Part model, mm, in its own coordinate system. A direction names the side the tool comes from. Give positions to 0.01 mm unless a question says otherwise; leave off trailing zeros. Order: outer loops, then holes, each group sorted by start corner. A loop starts at its lowest first (then second) coordinate and runs counter-clockwise, first axis right, second up. Notation, with made-up numbers: (66.25, 74) - (115.25, 74) arc R37 cw to (115.25, 111) - close; hole circle Ø4 at (86.5, 81). An arc over 180 degrees is marked (long way). One line per item, written item: value.
```python
from build123d import *

# Parameters (mm, degrees)
SKETCH1_W           = 2.4
SKETCH1_H           = 20
SKETCH1_H_2         = 2.4
SKETCH1_W_2         = 20
BOSS_EXTRUDE1_DEPTH = 20
BOSS_EXTRUDE2_DEPTH = 2.4
CUT_EXTRUDE1_REACH  = 4.4
SKETCH4_R           = 1.75
CUT_EXTRUDE2_REACH  = 4.4
SKETCH5_R           = 1.75
CUT_EXTRUDE3_REACH  = 24.4
SKETCH6_R           = 1.75
SKETCH7_R           = 2
BOSS_EXTRUDE3_DEPTH = 5
FILLET1_R           = 5


with BuildPart() as part:
    # Sketch1 → Boss-Extrude1 (new body)
    with BuildSketch(Plane(origin=(0, 0, 0), x_dir=(1, 0, 0), z_dir=(0, 1, 0))):
        with Locations((-1.2, 10)):
            Rectangle(SKETCH1_W, SKETCH1_H)
        with Locations((-1.2, -1.2)):
            Rectangle(SKETCH1_W, SKETCH1_H_2)
        with Locations((10, -1.2)):
            Rectangle(SKETCH1_W_2, SKETCH1_H_2)
    extrude(amount=-BOSS_EXTRUDE1_DEPTH)

    # Sketch2 → Boss-Extrude2 (add)
    with BuildSketch(Plane(origin=(0, 0, 0), x_dir=(1, 0, 0), z_dir=(0, 1, 0))):
        Polygon((20, -2.4), (20, 40), (0, 40), (0, 20), (-2.4, 20), (-2.4, -2.4), align=None)
    extrude(amount=BOSS_EXTRUDE2_DEPTH)

    # Sketch4 → Cut-Extrude1 (cut, up to next)
    with BuildSketch(Plane(origin=(0, 0, 0), x_dir=(0, 0, -1), z_dir=(1, 0, 0)), mode=Mode.PRIVATE) as cut_extrude1_sk1:
        with Locations((10, -10)):
            Circle(SKETCH4_R)
    cut_extrude1_tool1 = extrude(cut_extrude1_sk1.sketch, amount=-CUT_EXTRUDE1_REACH, mode=Mode.PRIVATE) & part.part
    add(cut_extrude1_tool1.solids().sort_by_distance((0, -10, -10))[0], mode=Mode.SUBTRACT)

    # Sketch5 → Cut-Extrude2 (cut, up to next)
    with BuildSketch(Plane(origin=(0, 0, 0), x_dir=(-1, 0, 0), z_dir=(0, 0, -1)), mode=Mode.PRIVATE) as cut_extrude2_sk1:
        with Locations((-10, -10)):
            Circle(SKETCH5_R)
    cut_extrude2_tool1 = extrude(cut_extrude2_sk1.sketch, amount=-CUT_EXTRUDE2_REACH, mode=Mode.PRIVATE) & part.part
    add(cut_extrude2_tool1.solids().sort_by_distance((10, -10, 0))[0], mode=Mode.SUBTRACT)

    # Sketch6 → Cut-Extrude3 (cut, up to next)
    with BuildSketch(Plane(origin=(0, 2.4, 0), x_dir=(1, 0, 0), z_dir=(0, 1, 0)), mode=Mode.PRIVATE) as cut_extrude3_sk1:
        with Locations((10, 30)):
            Circle(SKETCH6_R)
    cut_extrude3_tool1 = extrude(cut_extrude3_sk1.sketch, amount=-CUT_EXTRUDE3_REACH, mode=Mode.PRIVATE) & part.part
    add(cut_extrude3_tool1.solids().sort_by_distance((10, 2.4, -30))[0], mode=Mode.SUBTRACT)

    # Sketch7 → Boss-Extrude3 (add)
    with BuildSketch(Plane.XZ):
        with Locations((10, -10)):
            Circle(SKETCH7_R)
    extrude(amount=BOSS_EXTRUDE3_DEPTH)

    # Fillet1
    fillet1_edges = [part.edges().sort_by_distance(p)[0] for p in [
        (20, -20, 1.2),
        (20, 1.2, -40),
        (0, 1.2, -40),
        (-1.2, -20, -20),
    ]]
    fillet(fillet1_edges, radius=FILLET1_R)


solid = part.part
```
1) Cut at A-A, the plane y = -10. Give the cut face in (x, z), then the cut area to 3 significant figures.
Outcome:
outline: (-2.4, -20) - (0, -20) - (0, -11.75) - (-2.4, -11.75) - close; (-2.4, -8.25) - (0, -8.25) - (0, 0) - (8.25, 0) - (8.25, 2.4) - (-2.4, 2.4) - close; (11.75, 0) - (20, 0) - (20, 2.4) - (11.75, 2.4) - close
area: 85.0 mm^2
2) Mould opens along Z. For faces 3 (the cylindrical face through (19, 1, -38)), 4 (the cylindrical face through (-1.2, -8.5, -10.9)), 5 (the flat face through (10, -5, -10)) say: released by +Z, released by -Z, zero draft, split by the parting line, or undercut.
Outcome:
face 3: released by -Z
face 4: undercut
face 5: zero draft
3) Cut at D-D, the plane x = 6.5. Give the cut face in (y, z), then the cut area to 3 significant figures.
Outcome:
outline: (-20, 0) - (0, 0) - (0, -40) - (2.4, -40) - (2.4, 2.4) - (-20, 2.4) - close
area: 150 mm^2
4) Drill centre lines: line 1 along Y through (x, z) = (-1.15, -10); line 2 along X through (y, z) = (1.85, -30); line 3 along Z through (x, y) = (10, 1.35). Where is each one in solid material? Low to high. Write a range as from..to.
Outcome:
line 1: y = -20..-11.75, -8.25..2.4
line 2: x = 0..8.25, 11.75..20
line 3: z = -40..-31.75, -28.25..2.4
5) Cut at C-C, the plane x = 10. Give the cut face in (y, z).
Outcome:
outline: (-20, 0) - (-11.75, 0) - (-11.75, 2.4) - (-20, 2.4) - close; (-8.25, 0) - (0, 0) - (0, -8) - (-5, -8) - (-5, -12) - (0, -12) - (0, -28.25) - (2.4, -28.25) - (2.4, 2.4) - (-8.25, 2.4) - close; (0, -40) - (2.4, -40) - (2.4, -31.75) - (0, -31.75) - close
6) Cut at B-B, the plane z = -30. Give the cut face in (x, y).
Outcome:
outline: (0, 0) - (8.25, 0) - (8.25, 2.4) - (0, 2.4) - close; (11.75, 0) - (20, 0) - (20, 2.4) - (11.75, 2.4) - close
7) Which spindle directions (+Z, -Z, +X, -X, +Y, -Y) get a long thin tool onto all of the face, cutting with end or side? Do faces 1 (the flat face through (-0.2, -20, -3.1)), 2 (the flat face through (0, 1, -28)). Say none if no direction does.
Outcome:
face 1: +Z, -Z, +X, -X, -Y
face 2: -Z, -X, +Y, -Y
8) Pin check, flat tips, straight feed: pin 1 (0.7 mm diameter, centred on y = 1, z = -29.5, fed in from -X); pin 2 (10 mm diameter, centred on x = 12, z = -34, fed in from -Y); pin 3 (2.5 mm diameter, centred on x = -1.5, y = -7, fed in from -Z). Stop position of each tip, or through.
Outcome:
pin 1: stops at x = 0
pin 2: stops at y = 0
pin 3: stops at z = -20
